Geometry check sheet. Reference: the model listing, model coordinates, mm. Give positions to 0.01 mm unless a question says otherwise; leave off trailing zeros. Order: outer loops, then holes, each group sorted by start corner. A loop starts at its lowest first (then second) coordinate and runs counter-clockwise, first axis right, second up. Notation, with made-up numbers: M -18,-34 L 19,-34 A26 cw 19,-1 Z; hole C 48,-18 d3. An arc over 180 degrees is marked long. Answer as CSV lines item,"result".
from build123d import *

# Parameters (mm, degrees)
SKETCH1_W           = 63.5
SKETCH1_H           = 76.2
BOSS_EXTRUDE1_DEPTH = 914.4
SKETCH2_W           = 47.625
SKETCH2_H           = 60.325
CUT_EXTRUDE1_DEPTH  = 916.743977594
SKETCH3_R           = 7.9375
CUT_EXTRUDE2_DEPTH  = 918.393710465


with BuildPart() as part:
    # Sketch1 → Boss-Extrude1 (new body)
    with BuildSketch(Plane(origin=(0, 0, 0), x_dir=(1, 0, 0), z_dir=(0, 1, 0))):
        Rectangle(SKETCH1_W, SKETCH1_H)
    extrude(amount=BOSS_EXTRUDE1_DEPTH)

    # Sketch2 → Cut-Extrude1 (cut, through all)
    with BuildSketch(Plane(origin=(0, 914.4, 0), x_dir=(1, 0, 0), z_dir=(0, 1, 0))):
        Rectangle(SKETCH2_W, SKETCH2_H)
    extrude(amount=-CUT_EXTRUDE1_DEPTH, mode=Mode.SUBTRACT)

    # Sketch3 → Cut-Extrude2 (cut, through all)
    with BuildSketch(Plane(origin=(31.75, 0, 0), x_dir=(0, 0, -1), z_dir=(1, 0, 0))):
        with Locations((0, 311.15)):
            Circle(SKETCH3_R)
        with Locations((0, 133.35)):
            Circle(SKETCH3_R)
    extrude(amount=-CUT_EXTRUDE2_DEPTH, mode=Mode.SUBTRACT)


solid = part.part
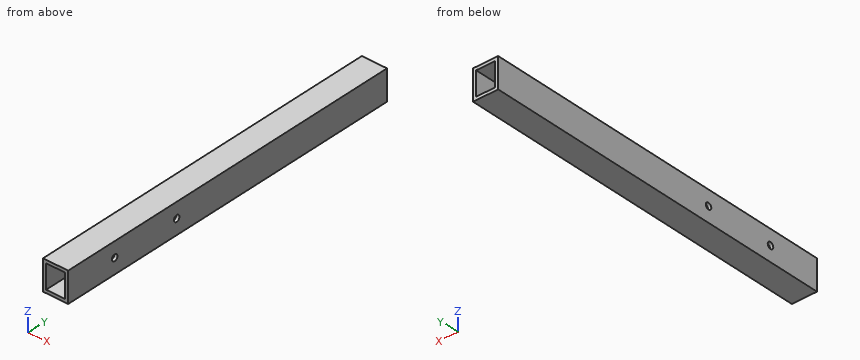
(1) Section check C-C on z = 0. Enter the section's corners in (x, y), then the cut area to 3 significant figures.
The answers:
outline,"M -31.75,0 L -23.81,0 L -23.81,125.41 L -31.75,125.41 Z; M -31.75,141.29 L -23.81,141.29 L -23.81,303.21 L -31.75,303.21 Z; M -31.75,319.09 L -23.81,319.09 L -23.81,914.4 L -31.75,914.4 Z; M 23.81,0 L 31.75,0 L 31.75,125.41 L 23.81,125.41 Z; M 23.81,141.29 L 31.75,141.29 L 31.75,303.21 L 23.81,303.21 Z; M 23.81,319.09 L 31.75,319.09 L 31.75,914.4 L 23.81,914.4 Z"
area,"14,000 mm2"
(2) Material ranges on line 1 (Y direction, x = 28, z = 0); line 2 (X direction, y = 342.5, z = 29); line 3 (Z direction, x = -14.5, y = 249.5), recorded low to high.
The answers:
line 1,"y = 0 to 125.41, 141.29 to 303.21, 319.09 to 914.4"
line 2,"x = -31.75 to -23.81, 23.81 to 31.75"
line 3,"z = -38.1 to -30.16, 30.16 to 38.1"
(3) Section check B-B on x = 5. Enter the section's corners in (y, z).
The answers:
outline,"M 0,-38.1 L 914.4,-38.1 L 914.4,-30.16 L 0,-30.16 Z; M 0,30.16 L 914.4,30.16 L 914.4,38.1 L 0,38.1 Z"
(4) Section check A-A on y = 133.35. Enter the section's corners in (x, z), then the cut area to 3 significant figures.
The answers:
outline,"M -31.75,-38.1 L 31.75,-38.1 L 31.75,-7.94 L 23.81,-7.94 L 23.81,-30.16 L -23.81,-30.16 L -23.81,-7.94 L -31.75,-7.94 Z; M -31.75,7.94 L -23.81,7.94 L -23.81,30.16 L 23.81,30.16 L 23.81,7.94 L 31.75,7.94 L 31.75,38.1 L -31.75,38.1 Z"
area,"1,710 mm2"
